Could you check a few things on this model? Use its own coordinates, in mm. A direction names the side the tool comes from. Coordinates: 2 decimals unless noted, no trailing zeros. Loops run counter-clockwise (first coordinate to the right, second up) from the corner with the lowest first, then second, coordinate; pieces in that order, holes last.
from build123d import *

# Parameters (mm, degrees)
BOSS_EXTRUDE1_DEPTH = 40
BOSS_EXTRUDE6_DEPTH = 40
CUT_EXTRUDE1_START  = 40
SKETCH9_W           = 55
SKETCH9_H           = 45
CUT_EXTRUDE1_DEPTH  = 38
CUT_EXTRUDE3_START  = 40
SKETCH10_W          = 32
SKETCH10_H          = 70
CUT_EXTRUDE3_DEPTH  = 38
FILLET4_R           = 2
SKETCH11_W          = 12
SKETCH11_H          = 36.5
CUT_EXTRUDE4_DEPTH  = 5


with BuildPart() as part:
    # Sketch1 → Boss-Extrude1 (new body)
    with BuildSketch(Plane(origin=(0, 0, 0), x_dir=(1, 0, 0), z_dir=(0, 1, 0))):
        with BuildLine():
            Line((38.137674452, -1.734509714), (-11.512325548, -1.734509714))
            ThreePointArc((-11.512325548, -1.734509714), (-16.285296321, -3.711538941), (-18.262325548, -8.484509714))
            Line((-18.262325548, -8.484509714), (-18.262325548, -58.134509714))
            ThreePointArc((-18.262325548, -58.134509714), (-14.234303537, -64.311348374), (-6.957633451, -63.116204195))
            Line((-6.957633451, -63.116204195), (-8.30717185, -61.640146571))
            ThreePointArc((-8.30717185, -61.640146571), (-16.222632836, -58.747294544), (-9.310805247, -53.925494584))
            Line((-9.310805247, -53.925494584), (-8.383849331, -52.153277687))
            ThreePointArc((-8.383849331, -52.153277687), (-11.302087657, -51.387784581), (-14.262325548, -51.970095711))
            Line((-14.262325548, -51.970095711), (-14.262325548, -12.660332986))
            ThreePointArc((-14.262325548, -12.660332986), (-15.047859454, -4.948975808), (-7.336502276, -5.734509714))
            Line((-7.336502276, -5.734509714), (31.973260449, -5.734509714))
            ThreePointArc((31.973260449, -5.734509714), (31.390949319, -8.694747605), (32.156442425, -11.612985931))
            Line((32.156442425, -11.612985931), (33.928659322, -10.686030015))
            ThreePointArc((33.928659322, -10.686030015), (38.750459282, -3.774202426), (41.643311309, -11.689663412))
            Line((41.643311309, -11.689663412), (43.119368933, -13.039201811))
            ThreePointArc((43.119368933, -13.039201811), (44.314513112, -5.762531725), (38.137674452, -1.734509714))
        make_face()
    extrude(amount=BOSS_EXTRUDE1_DEPTH)

    # Sketch8 → Boss-Extrude6 (add)
    with BuildSketch(Plane(origin=(0, 0, 0), x_dir=(1, 0, 0), z_dir=(0, 1, 0))):
        with BuildLine():
            Line((-18.262325548, -58.134509714), (-18.262325548, -8.484509714))
            ThreePointArc((-18.262325548, -8.484509714), (-16.285296321, -3.711538941), (-11.512325548, -1.734509714))
            Line((-11.512325548, -1.734509714), (38.137674452, -1.734509714))
            Line((38.137674452, -1.734509714), (38.137674452, 44.765490286))
            Line((38.137674452, 44.765490286), (-19.862325548, 44.765490286))
            Line((-19.862325548, 44.765490286), (-19.862325548, 14.865490286))
            Line((-19.862325548, 14.865490286), (-53.262325548, 14.865490286))
            Line((-53.262325548, 14.865490286), (-53.262325548, -58.134509714))
            Line((-53.262325548, -58.134509714), (-18.262325548, -58.134509714))
        make_face()
    extrude(amount=BOSS_EXTRUDE6_DEPTH)

    # Sketch9 → Cut-Extrude1 (cut)
    with BuildSketch(Plane(origin=(0, 0, 0), x_dir=(1, 0, 0), z_dir=(0, 1, 0)).offset(CUT_EXTRUDE1_START)):
        with Locations((9.137674452, 20.765490286)):
            Rectangle(SKETCH9_W, SKETCH9_H)
    extrude(amount=-CUT_EXTRUDE1_DEPTH, mode=Mode.SUBTRACT)

    # Sketch10 → Cut-Extrude3 (cut)
    with BuildSketch(Plane(origin=(0, 0, 0), x_dir=(1, 0, 0), z_dir=(0, 1, 0)).offset(CUT_EXTRUDE3_START)):
        with Locations((-35.681852139, -21.634509714)):
            Rectangle(SKETCH10_W, SKETCH10_H)
    extrude(amount=-CUT_EXTRUDE3_DEPTH, mode=Mode.SUBTRACT)

    # Fillet4
    fillet4_edges = [part.edges().sort_by_distance(p)[0] for p in [
        (-18.262325548, 20, 58.134509714),
        (38.137674452, 20, 1.734509714),
        (38.137674452, 20, -44.765490286),
        (-19.862325548, 20, -44.765490286),
        (-19.862325548, 20, -14.865490286),
        (-53.262325548, 20, -14.865490286),
        (-53.262325548, 20, 58.134509714),
    ]]
    fillet(fillet4_edges, radius=FILLET4_R)

    # Sketch11 → Cut-Extrude4 (cut)
    with BuildSketch(Plane(origin=(-18.362325548, 0, 0), x_dir=(0, 0, -1), z_dir=(1, 0, 0))):
        with Locations((4.265490286, 20.25)):
            Rectangle(SKETCH11_W, SKETCH11_H)
    extrude(amount=-CUT_EXTRUDE4_DEPTH, mode=Mode.SUBTRACT)


solid = part.part
(1) We'd pull the mould along Z, two halves only. Please class faces 4 (the face through (-36, 21, -13.365)), 5 (the face through (-36, 20, 58.135)), 6 (the face through (44.615, 19.72, 6.585)): +Z half, -Z half, draft (parallel to the pull), parting line (faces both ways), or undercut.
Answers:
face 4: undercut
face 5: +Z half
face 6: parting line
(2) Imagine slicing it at A-A, the plane z = -22. Write out the boundary of the cut face in (x, y).
Answers:
outline: (-19.86, 0) - (38.14, 0) - (38.14, 40) - (36.64, 40) - (36.64, 2) - (-18.36, 2) - (-18.36, 40) - (-19.86, 40) - close
(3) I need wall thicknesses on probe 1 along Z at (x, y) = (-32.5, 30); probe 2 along X at (y, z) = (18.5, -20.5); probe 3 along X at (y, z) = (35.5, -5). Which ranges of each line are inside material? Lowest first, please.
Answers:
probe 1: z = -14.87 to -13.37, 56.63 to 58.13
probe 2: x = -19.86 to -18.36, 36.64 to 38.14
probe 3: x = -53.26 to -51.68, 36.64 to 38.14
(4) Which directions (+Z, -Z, +X, -X, +Y, -Y) give clear straight access to the entire face, cutting with the end or side of a thin tool? Please do faces 1 (the face through (36.638, 21, -20)), 2 (the face through (-19.862, 20, -30)), 3 (the face through (-53.262, 20, 21)).
Answers:
face 1: +Y
face 2: -Z, -X, +Y, -Y
face 3: +Z, -Z, -X, +Y, -Y
(5) For pin 1 (12 mm diameter, centred on x = 12.5, y = 11.5, fed in from +Z); pin 2 (19 mm diameter, centred on y = 23, z = -18.5, fed in from +X); pin 3 (23.5 mm diameter, centred on x = -40, y = 16, fed in from -Z), each with a flat end and sliding along its axis, tell me the tip position at first contact or that it passes through.
Answers:
pin 1: stops at z = 5.73
pin 2: stops at x = 38.14
pin 3: stops at z = -14.87
(6) Imagine slicing it at C-C, the plane x = 3.5. Write out the boundary of the cut face in (y, z).
Answers:
outline: (0, -44.77) - (40, -44.77) - (40, -43.27) - (2, -43.27) - (2, 1.73) - (40, 1.73) - (40, 5.73) - (0, 5.73) - close
(7) Imagine slicing it at B-B, the plane x = -12. Write out the boundary of the cut face in (y, z), and give its area (3 significant figures).
Answers:
outline: (0, -44.77) - (40, -44.77) - (40, -43.27) - (2, -43.27) - (2, 1.73) - (40, 1.73) - (40, 3.51) - (0, 3.51) - close; (0, 51.4) - (40, 51.4) - (40, 53.41) - (0, 53.41) - close; (0, 62.86) - (40, 62.86) - (40, 64.87) - (0, 64.87) - close
area: 382 mm2
